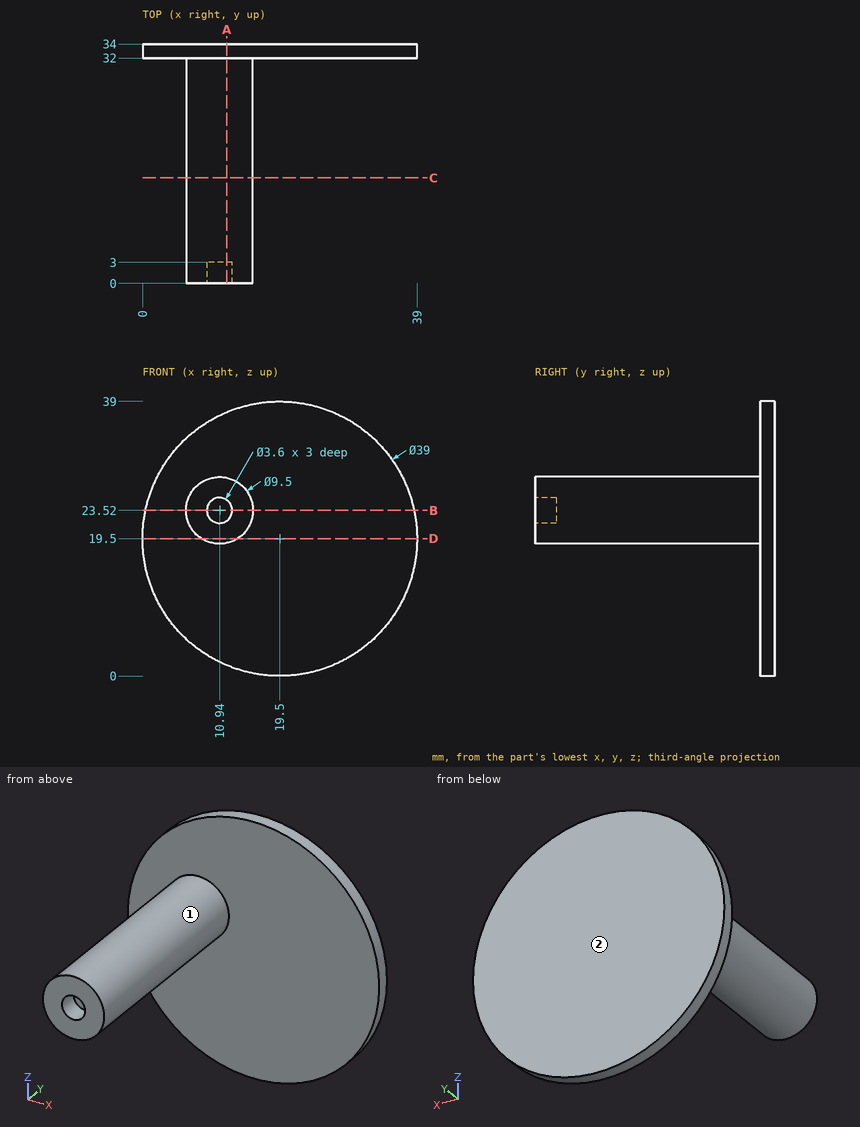
Design review of the part shown in the three views and the two pictorial views. Dimensions are in mm from the part's minimum x, y and z. A direction names the side the tool comes from. Round coordinates to 2 decimals unless told otherwise and drop trailing zeros. Loops run counter-clockwise (first coordinate to the right, second up) from the corner with the lowest first, then second, coordinate; pieces in that order, holes last. Notation, with made-up numbers: (81, 52.5) -> (88, 52.5) arc R19 cw to (88, 86.5) -> close; hole circle Ø2 at (54, 49.25). An arc over 180 degrees is marked (long way). Return JSON: item names as keys, results as strings.
(1) Add section A-A on x = 12. Write out the cut boundary in (y, z), plus the area to 3 significant figures.
Solved:
{"outline": "(0, 18.89) -> (32, 18.89) -> (32, 1.5) -> (34, 1.5) -> (34, 37.5) -> (32, 37.5) -> (32, 28.15) -> (0, 28.15) -> (0, 24.97) -> (3, 24.97) -> (3, 22.07) -> (0, 22.07) -> close", "area": "360 mm2"}
(2) For line 1 (Z direction, x = 10.94, y = 2.2); line 2 (Y direction, x = 34, z = 9.5); line 3 (Z direction, x = 15, y = 31), list the stretches that pass through material, from the lowest coordinate up.
Solved:
{"line 1": "18.77 to 21.72, 25.32 to 28.27", "line 2": "32 to 34", "line 3": "21.05 to 25.99"}
(3) For the marked faces 1 and 2, list the 3-axis set-ups (+Z, -Z, +X, -X, +Y, -Y) from which the entire face can be reached by the end or side of a thin tool; tool diameter is ignored.
Solved:
{"face 1": "-Y", "face 2": "+Z, -Z, +X, -X, +Y"}
(4) Add section B-B on z = 23.52. Write out the cut boundary in (x, y), plus the area to 3 significant figures.
Solved:
{"outline": "(0.42, 32) -> (6.19, 32) -> (6.19, 0) -> (9.14, 0) -> (9.14, 3) -> (12.74, 3) -> (12.74, 0) -> (15.69, 0) -> (15.69, 32) -> (38.58, 32) -> (38.58, 34) -> (0.42, 34) -> close", "area": "370 mm2"}
(5) For pin 1 (1.8 mm diameter, centred on x = 10.5, z = 24, fed in from -Y); pin 2 (12 mm diameter, centred on y = 7, z = 11.5, fed in from +X); pin 3 (1.5 mm diameter, centred on y = 29, z = 20.5, fed in from -X); pin 4 (3 mm diameter, centred on y = 7, z = 18, fed in from +X), all flat-tipped, find the tip position at first contact; note any pin that passes through.
Solved:
{"pin 1": "y = 3", "pin 2": "through", "pin 3": "x = 6.77", "pin 4": "x = 13.47"}
(6) Add section D-D on z = 19.5. Write out the cut boundary in (x, y), plus the area to 3 significant figures.
Solved:
{"outline": "(0, 32) -> (8.41, 32) -> (8.41, 0) -> (13.47, 0) -> (13.47, 32) -> (39, 32) -> (39, 34) -> (0, 34) -> close", "area": "240 mm2"}
(7) Add section C-C on y = 15. Write out the cut boundary in (x, z).
Solved:
{"outline": "circle Ø9.5 at (10.94, 23.52)"}
